Work out the finished part from the listing and answer in its coordinate system (mm). Round coordinates to 2 decimals unless told otherwise and drop trailing zeros. Loops run counter-clockwise (first coordinate to the right, second up) from the corner with the lowest first, then second, coordinate; pieces in that order, holes last.
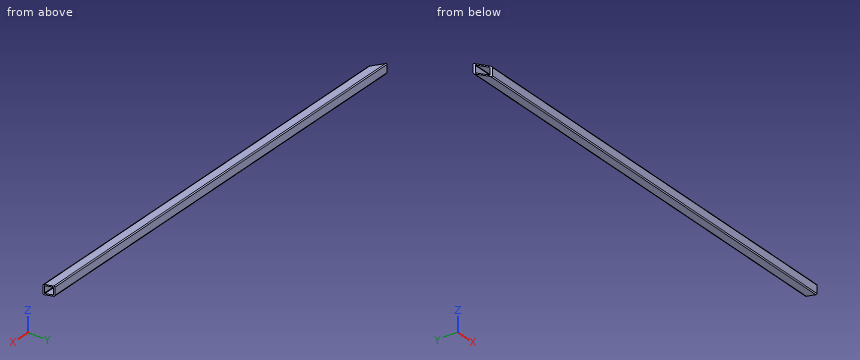
```python
from build123d import *

# Parameters (mm, degrees)
SKETCH3_W           = 25.4
SKETCH3_H           = 25.4
SKETCH3_W_2         = 19.304
SKETCH3_H_2         = 19.304
BOSS_EXTRUDE1_DEPTH = 1190.03
FILLET1_R           = 2.5
FILLET2_R           = 1
CUT_EXTRUDE1_DEPTH  = 1191.368787771


with BuildPart() as part:
    # Sketch3 → Boss-Extrude1 (new body)
    with BuildSketch(Plane(origin=(0, 0, 0), x_dir=(0, 0, -1), z_dir=(1, 0, 0))):
        Rectangle(SKETCH3_W, SKETCH3_H)
        Rectangle(SKETCH3_W_2, SKETCH3_H_2, mode=Mode.SUBTRACT)
    extrude(amount=-BOSS_EXTRUDE1_DEPTH)

    # Fillet1
    fillet1_edges = [part.edges().sort_by_distance(p)[0] for p in [
        (-595.015, -12.7, -12.7),
        (-595.015, -12.7, 12.7),
        (-595.015, 12.7, 12.7),
        (-595.015, 12.7, -12.7),
    ]]
    fillet(fillet1_edges, radius=FILLET1_R)

    # Fillet2
    fillet2_edges = [part.edges().sort_by_distance(p)[0] for p in [
        (-595.015, 9.652, -9.652),
        (-595.015, -9.652, -9.652),
        (-595.015, -9.652, 9.652),
        (-595.015, 9.652, 9.652),
    ]]
    fillet(fillet2_edges, radius=FILLET2_R)

    # Sketch5 → Cut-Extrude1 (cut, through all)
    with BuildSketch(Plane(origin=(0, 0, -12.7), x_dir=(-1, 0, 0), z_dir=(0, 0, -1))):
        Polygon((1190.03, 12.7), (1155.06989922, -12.7), (1190.03, -12.7), align=None)
        Polygon((0, 12.7), (8.252960284, 12.7), (0, -12.7), align=None)
    extrude(amount=-CUT_EXTRUDE1_DEPTH, mode=Mode.SUBTRACT)


solid = part.part
```
1. Consider probe 1 along Y at (x, z) = (-56, 4.5); probe 2 along Y at (x, z) = (-475.5, -9). Determine where each line is inside the solid, lowest interval first.
Answer key:
probe 1: y = -12.7 to -9.65, 9.65 to 12.7
probe 2: y = -12.7 to -9.59, 9.59 to 12.7
2. Given pin 1 (10 mm diameter, centred on y = 1.5, z = -0.5, fed in from -X), flat-ended and moving along its own axis, determine where the tip first touches the part or whether it passes through.
Answer key:
pin 1: passes through
3. Find section A-A (z = 1.75). Write down the section's boundary in (x, y).
Answer key:
outline: (-1190.03, 12.7) - (-1185.83, 9.65) - (-7.26, 9.65) - (-8.25, 12.7) - close; (-1159.27, -9.65) - (-1155.07, -12.7) - (0, -12.7) - (-0.99, -9.65) - close
4. Find section C-C (x = -129). Write down the section's boundary in (y, z), then the cut area to 3 significant figures.
Answer key:
outline: (-12.7, -10.2) arc R2.5 ccw to (-10.2, -12.7) - (10.2, -12.7) arc R2.5 ccw to (12.7, -10.2) - (12.7, 10.2) arc R2.5 ccw to (10.2, 12.7) - (-10.2, 12.7) arc R2.5 ccw to (-12.7, 10.2) - close; hole (-9.65, -8.65) arc R1 ccw to (-8.65, -9.65) - (8.65, -9.65) arc R1 ccw to (9.65, -8.65) - (9.65, 8.65) arc R1 ccw to (8.65, 9.65) - (-8.65, 9.65) arc R1 ccw to (-9.65, 8.65) - close
area: 268 mm2
5. Find section B-B (y = -4.25). Write down the section's boundary in (x, z).
Answer key:
outline: (-1166.7, -12.7) - (-2.75, -12.7) - (-2.75, -9.65) - (-1166.7, -9.65) - close; (-1166.7, 9.65) - (-2.75, 9.65) - (-2.75, 12.7) - (-1166.7, 12.7) - close
